Here's how the part is built. I have some questions about the finished solid (model axes, mm). A direction names the side the tool comes from. Give positions to 0.01 mm unless a question says otherwise; leave off trailing zeros. Loops run counter-clockwise (first coordinate to the right, second up) from the corner with the lowest first, then second, coordinate; pieces in that order, holes last. Notation, with made-up numbers: (-36, 39) -> (-25, 39) arc R31 ccw to (-25, 78) -> close; hole circle Ø4 at (14.5, 8.5). An arc over 180 degrees is marked (long way). Answer in a Markdown table with one row per item. Add a question column.
Item 1: If I drill on line 1 (Z direction, x = -5, y = -36.9); line 2 (Z direction, x = -7.25, y = -38.3); line 3 (Y direction, x = -0.75, z = 88.25), over which ranges is the centre line in solid material (lowest first)?
Item 2: If we section it at D-D (z = 70.25): Write out the boundary of the cut face in (x, y), then the cut area to 3 significant figures.
Item 3: For P1, Ø6, axis at x = -9, z = 79.5, coming from the -Y side; P2, Ø4, axis at x = -7, z = 71.5, coming from the +Y side; P3, Ø2, axis at x = -3, z = 76, coming from the -Y side; P4, Ø2, axis at x = -3, z = 66, coming from the -Y side, each with a flat end and sliding along its axis, tell me the tip position at first contact or that it passes through.
Item 4: If we section it at B-B (x = -1.5): Write out the boundary of the cut face in (y, z).
Item 5: Which directions (+Z, -Z, +X, -X, +Y, -Y) give clear straight access to the entire face, cutting with the end or side of a thin tool? Please do faces 1 (the face through (0, -40.4, 78.5)), 2 (the face through (-5, -36.48, 91)), 3 (the face through (-5, -36.48, 66)).
Item 6: If we section it at A-A (y = -39.65): Write out the boundary of the cut face in (x, z).
Item 7: If we section it at C-C (y = -36.85): Write out the boundary of the cut face in (x, z).
```python
from build123d import *

# Parameters (mm, degrees)
BOSS_EXTRU_1_DEPTH = 10


with BuildPart() as part:
    # Esquisse1 → Boss.-Extru.1 (new body)
    with BuildSketch(Plane(origin=(0, 0, 0), x_dir=(0, 0, -1), z_dir=(1, 0, 0))):
        with BuildLine():
            Line((-89.898468063, -36.480057998), (-91.898468063, -36.480057998))
            Line((-91.898468063, -36.480057998), (-91.898468063, -35.480057998))
            Line((-91.898468063, -35.480057998), (-89.475592066, -35.480057998))
            ThreePointArc((-89.475592066, -35.480057998), (-78.569905432, -40.181223159), (-67.664218798, -35.480057998))
            Line((-67.664218798, -35.480057998), (-65.241342801, -35.480057998))
            Line((-65.241342801, -35.480057998), (-65.241342801, -36.480057998))
            Line((-65.241342801, -36.480057998), (-67.241342801, -36.480057998))
            ThreePointArc((-67.241342801, -36.480057998), (-78.569905432, -41.181223159), (-89.898468063, -36.480057998))
        make_face()
    extrude(amount=-BOSS_EXTRU_1_DEPTH)


solid = part.part
```
Recorded:
| question | item | result |
|---|---|---|
| 1 | line 1 | z = 67.68 to 69.21, 87.93 to 89.46 |
| 1 | line 2 | z = 69.41 to 71.3, 85.84 to 87.73 |
| 1 | line 3 | y = -37.92 to -36.64 |
| 2 | outline | (-10, -38.85) -> (0, -38.85) -> (0, -37.66) -> (-10, -37.66) -> close |
| 2 | area | 11.9 mm^2 |
| 3 | P1 | stops at y = -41.18 |
| 3 | P2 | stops at y = -37.13 |
| 3 | P3 | stops at y = -41.1 |
| 3 | P4 | stops at y = -36.48 |
| 4 | outline | (-36.48, 65.24) -> (-35.48, 65.24) -> (-35.48, 67.66) arc R15 cw to (-35.48, 89.48) -> (-35.48, 91.9) -> (-36.48, 91.9) -> (-36.48, 89.9) arc R16 ccw to (-36.48, 67.24) -> close |
| 5 | face 1 | +Z, -Z, +X, +Y, -Y |
| 5 | face 2 | +Z, +X, -X, -Y |
| 5 | face 3 | -Z, +X, -X, -Y |
| 6 | outline | (-10, 71.74) -> (0, 71.74) -> (0, 74.61) -> (-10, 74.61) -> close; (-10, 82.53) -> (0, 82.53) -> (0, 85.4) -> (-10, 85.4) -> close |
| 7 | outline | (-10, 67.62) -> (0, 67.62) -> (0, 69.14) -> (-10, 69.14) -> close; (-10, 88) -> (0, 88) -> (0, 89.52) -> (-10, 89.52) -> close |
